from build123d import *

# Parameters (mm, degrees)
F0_R     = 3
F1_DEPTH = 14
F3_DEPTH = 25
F4_R     = 1
F5_DEPTH = 20.001


with BuildPart() as f1:
    # F0 (on Front) → F1 (new body)
    with BuildSketch(Plane.XZ):
        Polygon((21, 20), (-21, 20), (-21, 14), (-9, 14), (-9, -17.5), (9, -17.5), (9, 14), (21, 14), align=None)
        Circle(F0_R, mode=Mode.SUBTRACT)
    extrude(amount=F1_DEPTH)

    # F2 (on Front) → F3 (cut)
    with BuildSketch(Plane.XZ):
        with BuildLine():
            Line((-1, -17.5), (1, -17.5))
            Line((1, -17.5), (1, -2.828427))
            ThreePointArc((1, -2.828427), (0, -3), (-1, -2.828427))
            Line((-1, -2.828427), (-1, -17.5))
        make_face()
    extrude(amount=F3_DEPTH, mode=Mode.SUBTRACT)

    # F4 (on Top) → F5 (cut, through all)
    with BuildSketch(Plane.XY):
        with Locations((-16, -7)):
            Circle(F4_R)
        with BuildLine():
            ThreePointArc((17, -7), (16, -6), (15, -7))
            ThreePointArc((15, -7), (16, -8), (17, -7))
        make_face()
    extrude(amount=F5_DEPTH, mode=Mode.SUBTRACT)


solid = f1.part
Part model, mm, in its own coordinate system. A direction names the side the tool comes from. Round coordinates to 2 decimals unless told otherwise and drop trailing zeros. Order: outer loops, then holes, each group sorted by start corner. A loop starts at its lowest first (then second) coordinate and runs counter-clockwise, first axis right, second up. Notation, with made-up numbers: (-39, 59.5) -> (-13, 59.5) arc R28 ccw to (-13, 79.5) -> close; hole circle Ø11 at (65.5, 66). An arc over 180 degrees is marked (long way). Put each result on its own line as item: value.
Q1. Wall check: line 1 (X direction, y = -1.75, z = -9.5); line 2 (Y direction, x = -16, z = 16.35); line 3 (X direction, y = -10.5, z = 0). Give the ranges that are in metal, low to high. Write a range as [from, to].
From the geometry:
line 1: x = [-9, -1], [1, 9]
line 2: y = [-14, -8], [-6, 0]
line 3: x = [-9, -3], [3, 9]
Q2. Tool access for faces 5 (the face through (1, -7, -10)), 6 (the face through (14, -7, 14)), 7 (the face through (-14, -7, 14)), 8 (the face through (-5, -7, -17.5)): list every direction of +Z, -Z, +X, -X, +Y, -Y with a clear straight run to the whole face (end or side of a thin tool).
From the geometry:
face 5: -Z, +Y, -Y
face 6: -Z, +X, +Y, -Y
face 7: -Z, -X, +Y, -Y
face 8: -Z, +X, -X, +Y, -Y
Q3. Pull direction Y, two halves, no side cores. Call faces 1 (the face through (0, 0, 10)), 2 (the face through (0, -14, 10)), 3 (the face through (-15, -7, 17)), 4 (the face through (21, -7, 17)): pulls with the +Y half, pulls with the -Y half, needs draft (parallel to the pull), parting line crosses it, or undercut.
From the geometry:
face 1: pulls with the +Y half
face 2: pulls with the -Y half
face 3: undercut
face 4: needs draft
Q4. Band-saw the part on D-D (y = -11.75). Give the cut face in (x, z).
From the geometry:
outline: (-21, 14) -> (-9, 14) -> (-9, -17.5) -> (-1, -17.5) -> (-1, -2.83) arc R3 cw (long way) to (1, -2.83) -> (1, -17.5) -> (9, -17.5) -> (9, 14) -> (21, 14) -> (21, 20) -> (-21, 20) -> close
Q5. Band-saw the part on B-B (z = -10.5). Give the cut face in (x, y).
From the geometry:
outline: (-9, -14) -> (-1, -14) -> (-1, 0) -> (-9, 0) -> close; (1, -14) -> (9, -14) -> (9, 0) -> (1, 0) -> close
Q6. Band-saw the part on A-A (x = 16). Give the cut face in (y, z).
From the geometry:
outline: (-14, 14) -> (-8, 14) -> (-8, 20) -> (-14, 20) -> close; (-6, 14) -> (0, 14) -> (0, 20) -> (-6, 20) -> close
Q7. Band-saw the part on C-C (y = -7). Give the cut face in (x, z).
From the geometry:
outline: (-21, 14) -> (-17, 14) -> (-17, 20) -> (-21, 20) -> close; (-15, 14) -> (-9, 14) -> (-9, -17.5) -> (-1, -17.5) -> (-1, -2.83) arc R3 cw (long way) to (1, -2.83) -> (1, -17.5) -> (9, -17.5) -> (9, 14) -> (15, 14) -> (15, 20) -> (-15, 20) -> close; (17, 14) -> (21, 14) -> (21, 20) -> (17, 20) -> close
Q8. Pin check, flat tips, straight feed: pin 1 Ø12 at (x, z) = (6.5, -13.5) entering from +Y; pin 2 Ø5 at (y, z) = (-3.5, -1) entering from -X; pin 3 Ø1 at (y, z) = (-9.5, -7) entering from +X; pin 4 Ø2 at (x, y) = (-14, -6) entering from -Z. Stop position of each tip, or through.
From the geometry:
pin 1: stops at y = 0
pin 2: stops at x = -9
pin 3: stops at x = 9
pin 4: stops at z = 14
